Design review of the part built by this model. Coordinates are the model's own, in mm. Coordinates: 2 decimals unless noted, no trailing zeros. Loops run counter-clockwise (first coordinate to the right, second up) from the corner with the lowest first, then second, coordinate; pieces in that order, holes last. Notation, with made-up numbers: (14, 51) -> (61, 51) arc R27 ccw to (61, 85) -> close; hole circle Ø3 at (49.5, 87.5). An arc over 180 degrees is marked (long way). One line per item, written item: value. Start each with the question number.
1. Add section A-A on z = 2.25. Write out the cut boundary in (x, y) (3 decimals).
2. Add section B-B on y = 2.2. Write out the cut boundary in (x, z) (3 decimals), plus the area to 3 significant figures.
3. Add section D-D on x = -51.5. Write out the cut boundary in (y, z) (3 decimals).
4. For probe 1 along Z at (x, y) = (-19, 2.55); probe 2 along X at (y, z) = (0.7, 6.25) (3 decimals); probe 3 along X at (y, z) = (1.25, -0.25) (3 decimals), list the stretches that pass through material, from the lowest coordinate up.
5. Add section C-C on x = 71. Write out the cut boundary in (y, z) (3 decimals).
6. Insertion check: pin 1 (1.6 mm diameter, centred on x = 95, y = 1.5, fed in from -Z); pin 2 (1.5 mm diameter, centred on x = -11.5, y = 1.5, fed in from +Z); pin 3 (1 mm diameter, centred on y = 1.5, z = -5.5, fed in from -X); pin 4 (2 mm diameter, centred on x = 47.6, z = -0.65, fed in from +Y). Each pin has a flat end and moves straight along its axis. Give the tip position at first contact, or say it passes through.
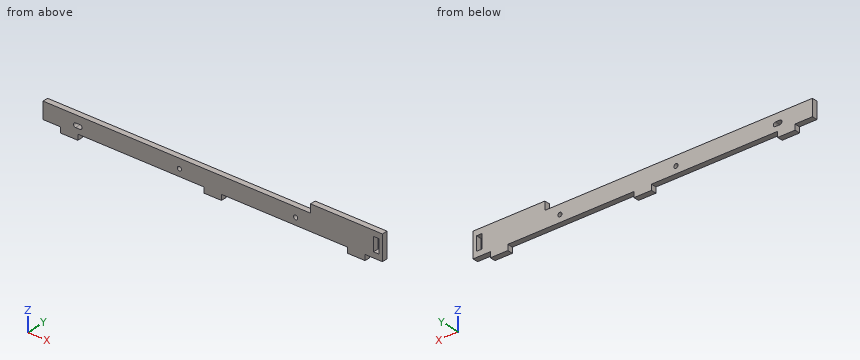
```python
from build123d import *

# Parameters (mm, degrees)
SKETCH1_W                = 195
SKETCH1_H                = 9.5
BOSS_EXTRUDE1_DEPTH      = 3.175
M2_CLEARANCE_HOLE1_D     = 2.4
SKETCH5_W                = 10
SKETCH5_H                = 3.175
BOSS_EXTRUDE2_DEPTH      = 3.175
SKETCH6_W                = 41.3
SKETCH6_H                = 3.175
BOSS_EXTRUDE3_DEPTH      = 4.8
SKETCH7_W                = 3.175
SKETCH7_H                = 8
CUT_EXTRUDE1_DEPTH       = 99.01802449
M2_CLEARANCE_SLOT1_DEPTH = 3.175


# Read off the part's stored shape, not the designer's step: M2 Clearance Slot1
with BuildPart() as part:
    # Sketch1 → Boss-Extrude1 (new body)
    with BuildSketch(Plane(origin=(0, 0, 0), x_dir=(1, 0, 0), z_dir=(0, 1, 0))):
        Rectangle(SKETCH1_W, SKETCH1_H)
    extrude(amount=BOSS_EXTRUDE1_DEPTH)

    # M2 Clearance Hole1 (through all)
    with Locations(Plane(origin=(0, 3.175, 0), x_dir=(1, 0, 0), z_dir=(0, 1, 0))):
        with Locations((-77.5, 0.65), (47.6, 0.65), (-19.1, 0.65)):
            Hole(M2_CLEARANCE_HOLE1_D / 2)

    # Sketch5 → Boss-Extrude2 (add)
    with BuildSketch(Plane(origin=(0, 0, -4.75), x_dir=(-1, 0, 0), z_dir=(0, 0, -1))):
        with Locations((82.5, 1.5875)):
            Rectangle(SKETCH5_W, SKETCH5_H)
        with Locations((-82.5, 1.5875)):
            Rectangle(SKETCH5_W, SKETCH5_H)
        with Locations((0, 1.5875)):
            Rectangle(SKETCH5_W, SKETCH5_H)
    extrude(amount=BOSS_EXTRUDE2_DEPTH)

    # Sketch6 → Boss-Extrude3 (add)
    with BuildSketch(Plane.XY.offset(4.75)):
        with Locations((76.85, 1.5875)):
            Rectangle(SKETCH6_W, SKETCH6_H)
    extrude(amount=BOSS_EXTRUDE3_DEPTH)

    # Sketch7 → Cut-Extrude1 (cut, through all)
    with BuildSketch(Plane(origin=(0, 3.175, 0), x_dir=(1, 0, 0), z_dir=(0, 1, 0))):
        with Locations((93.8875, -2.4)):
            Rectangle(SKETCH7_W, SKETCH7_H)
    extrude(amount=-CUT_EXTRUDE1_DEPTH, mode=Mode.SUBTRACT)

    # M2 Clearance Slot1 outline → M2 Clearance Slot1 (cut)
    with BuildSketch(Plane(origin=(0, 0, 0), x_dir=(1, 0, 0), z_dir=(0, 1, 0))):
        with BuildLine():
            ThreePointArc((-78.8, 1.85), (-80, 0.65), (-78.8, -0.55))
            Line((-78.8, -0.55), (-77.5, -0.55))
            ThreePointArc((-77.5, -0.55), (-78.7, 0.65), (-77.5, 1.85))
            Line((-77.5, 1.85), (-78.8, 1.85))
        make_face()
        with BuildLine():
            ThreePointArc((-77.5, 1.85), (-76.3, 0.65), (-77.5, -0.55))
            Line((-77.5, -0.55), (-76.2, -0.55))
            ThreePointArc((-76.2, -0.55), (-75, 0.65), (-76.2, 1.85))
            Line((-76.2, 1.85), (-77.5, 1.85))
        make_face()
    extrude(amount=M2_CLEARANCE_SLOT1_DEPTH, mode=Mode.SUBTRACT)


solid = part.part
```
Worked answers:
1. outline: (-97.5, 0) -> (92.3, 0) -> (92.3, 3.175) -> (-97.5, 3.175) -> close; (95.475, 0) -> (97.5, 0) -> (97.5, 3.175) -> (95.475, 3.175) -> close
2. outline: (-97.5, -4.75) -> (-87.5, -4.75) -> (-87.5, -7.925) -> (-77.5, -7.925) -> (-77.5, -4.75) -> (-5, -4.75) -> (-5, -7.925) -> (5, -7.925) -> (5, -4.75) -> (77.5, -4.75) -> (77.5, -7.925) -> (87.5, -7.925) -> (87.5, -4.75) -> (97.5, -4.75) -> (97.5, 9.55) -> (56.2, 9.55) -> (56.2, 4.75) -> (-97.5, 4.75) -> close; hole (-78.8, -1.85) -> (-76.2, -1.85) arc R1.2 ccw to (-76.2, 0.55) -> (-78.8, 0.55) arc R1.2 ccw to start; hole circle Ø2.4 at (-19.1, -0.65); hole circle Ø2.4 at (47.6, -0.65); hole (92.3, -1.6) -> (95.475, -1.6) -> (95.475, 6.4) -> (92.3, 6.4) -> close
2. area: 2,100 mm²
3. outline: (0, -4.75) -> (3.175, -4.75) -> (3.175, 4.75) -> (0, 4.75) -> close
4. probe 1: z = -4.75 to -1.85, 0.55 to 4.75
4. probe 2: x = 56.2 to 92.3, 95.475 to 97.5
4. probe 3: x = -97.5 to -79.931, -75.069 to -20.231, -17.969 to 46.469, 48.731 to 92.3, 95.475 to 97.5
5. outline: (0, -4.75) -> (3.175, -4.75) -> (3.175, 9.55) -> (0, 9.55) -> close
6. pin 1: stops at z = -4.75
6. pin 2: stops at z = 4.75
6. pin 3: stops at x = -87.5
6. pin 4: passes through
